Read the model definition and answer for the solid it produces. Units are mm, in the model's axes. Coordinates: 2 decimals unless noted, no trailing zeros. Write each loop counter-clockwise with the first axis right and the second up, starting at its lowest first coordinate (ties: lowest second). Pieces come first, ordered by that corner, then holes. Notation, with made-up numbers: (81, 83.25) -> (109, 83.25) arc R32 cw to (109, 115.25) -> close; hole circle Ø5 at (-12.5, 42). An arc over 180 degrees is marked (long way). Answer as a JSON object with one key per item and string values. Group by question number.
(1) Find section A-A (x = 0). Give the vertices of the cut face in (y, z) (1 decimal).
(2) Find section D-D (x = 33.5). Give the vertices of the cut face in (y, z) (3 decimals), then the cut area to 3 significant figures.
(3) Straight lines are drawn through the part: L1, parallel to X at y = -2, z = 2.65; L2, parallel to Y at x = -5, z = 2; L3, parallel to Y at x = 87.5, z = 3.05. For each, find the intervals that lie inside material, in ascending order.
(4) Find section B-B (z = 2.65). Count the separate pieces of the cut face and the enclosed holes in it, then the cut area to 3 significant figures.
(5) Find section C-C (y = -163.5). Give the vertices of the cut face in (x, z) (3 decimals), then the cut area to 3 significant figures.
(6) For a pull along X with two mould halves and no side action, classify faces 1 (the face through (59.7, -190.8, 1.6)), 2 (the face through (90.73, -233.17, 1.57)), 3 (the face through (-40.3, 31.69, 1.57)) as +X half, -X half, draft (parallel to the pull), parting line (faces both ways), or undercut.
(7) A flat-ended cylindrical pin translates along its axis: P1, Ø20.5, axis at x = 87.31, y = -238.52, coming from the -Z side. Find the tip coordinate at first contact, or state that the pin passes through.
from build123d import *

# Parameters (mm, degrees)
SKETCH1_R           = 6.35
SKETCH1_R_2         = 4.7244
SKETCH1_R_3         = 14.2875
BOSS_EXTRUDE1_DEPTH = 3.175
SKETCH2_R           = 10.16
SKETCH2_R_2         = 9.525
BOSS_EXTRUDE2_DEPTH = 3.175
BOSS_EXTRUDE3_DEPTH = 3.175


with BuildPart() as part:
    # Sketch1 → Boss-Extrude1 (new body)
    with BuildSketch(Plane.XY):
        with BuildLine():
            Line((123.825, 9.525), (50.373687682, 9.525))
            ThreePointArc((50.373687682, 9.525), (-42.021955485, 29.366465449), (8.37139721, -50.578194358))
            Line((8.37139721, -50.578194358), (78.367942069, -241.795763571))
            ThreePointArc((78.367942069, -241.795763571), (88.258712803, -247.99942994), (96.727824138, -239.962827716))
            Line((96.727824138, -239.962827716), (133.240324138, -1.441282895))
            ThreePointArc((133.240324138, -1.441282895), (131.051819652, 6.204732284), (123.825, 9.525))
        make_face()
        with Locations((87.3125, -238.521544821)):
            Circle(SKETCH1_R, mode=Mode.SUBTRACT)
        with Locations((123.825, 0)):
            Circle(SKETCH1_R_2, mode=Mode.SUBTRACT)
        Circle(SKETCH1_R_3, mode=Mode.SUBTRACT)
    extrude(amount=BOSS_EXTRUDE1_DEPTH)

    # Sketch2 → Boss-Extrude2 (add)
    with BuildSketch(Plane(origin=(0, 0, 0), x_dir=(-1, 0, 0), z_dir=(0, 0, -1))):
        with Locations((-87.3125, -238.521544821)):
            Circle(SKETCH2_R)
        with Locations((-87.3125, -238.521544821)):
            Circle(SKETCH2_R_2, mode=Mode.SUBTRACT)
    extrude(amount=-BOSS_EXTRUDE2_DEPTH)

    # Sketch3 → Boss-Extrude3 (add)
    with BuildSketch(Plane(origin=(0, 0, 0), x_dir=(-1, 0, 0), z_dir=(0, 0, -1))):
        with BuildLine():
            ThreePointArc((-50.373687682, 9.525), (-39.281923062, 32.941835958), (-18.155694858, 47.943766852))
            Line((-18.155694858, 47.943766852), (-123.825, 9.525))
            Line((-123.825, 9.525), (-50.373687682, 9.525))
        make_face()
        with BuildLine():
            Line((-8.37139721, -50.578194358), (-42.762000357, -144.526939268))
            Line((-42.762000357, -144.526939268), (41.245405611, -30.447504852))
            ThreePointArc((41.245405611, -30.447504852), (19.273979145, -47.505239328), (-8.37139721, -50.578194358))
        make_face()
    extrude(amount=-BOSS_EXTRUDE3_DEPTH)


solid = part.part
Results below:
{
 "1": {"outline": "(-86.5, 0) -> (-14.3, 0) -> (-14.3, 3.2) -> (-86.5, 3.2) -> close; (14.3, 0) -> (51.3, 0) -> (51.3, 3.2) -> (14.3, 3.2) -> close"},
 "2": {"outline": "(-131.949, 0) -> (42.365, 0) -> (42.365, 3.175) -> (-131.949, 3.175) -> close", "area": "553 mm2"},
 "3": {"L1": "x = -51.23 to -14.15, 14.15 to 119.54, 128.11 to 133.15", "L2": "y = -79.67 to -13.38, 13.38 to 51.02", "L3": "y = -248.68 to -244.87, -232.17 to 22.73"},
 "4": {"separate pieces": "1", "enclosed holes": "3", "area": "28,600 mm2"},
 "5": {"outline": "(49.707, 0) -> (108.433, 0) -> (108.433, 3.175) -> (49.707, 3.175) -> close", "area": "186 mm2"},
 "6": {"face 1": "-X half", "face 2": "undercut", "face 3": "parting line"},
 "7": {"P1": "stops at z = 0"}
}
